Check sheet for the modelled part. Datum: model origin and axes. Units: mm. Coordinates: 2 decimals unless noted, no trailing zeros. Write each loop counter-clockwise with the first axis right and the second up, starting at its lowest first coordinate (ties: lowest second). Pieces come first, ordered by that corner, then holes. Notation, with made-up numbers: (62, 21.5) -> (120, 21.5) arc R36 cw to (120, 55.5) -> close; hole circle Ø8 at (47.25, 37.25). An arc over 180 degrees is marked (long way). Put each result on its own line as item: value.
```python
from build123d import *

# Parameters (mm, degrees)
MODEL_R             = 2.5
MODEL_W             = 7.5
MODEL_H             = 60.000012028
BOSS_EXTRUDE1_DEPTH = 6.35


with BuildPart() as part:
    # Model → Boss-Extrude1 (new body)
    with BuildSketch(Plane.XY):
        Polygon((691.840616937, 302.611489719), (346.840616937, 302.611489719), (346.840616937, 367.611489719), (368.840616937, 367.611489719), (368.840616937, 447.611489719), (345.840616937, 447.611489719), (345.840616937, 534.611489719), (368.840616937, 534.611489719), (368.840616937, 644.611489719), (691.840616937, 644.611489719), align=None)
        with Locations((355.840616937, 514.611489719)):
            Circle(MODEL_R, mode=Mode.SUBTRACT)
        with Locations((355.840616937, 492.611489719)):
            Circle(MODEL_R, mode=Mode.SUBTRACT)
        with Locations((355.840616937, 467.611489719)):
            Circle(MODEL_R, mode=Mode.SUBTRACT)
        with Locations((356.840616937, 347.611489719)):
            Circle(MODEL_R, mode=Mode.SUBTRACT)
        with Locations((356.840616937, 322.611489719)):
            Circle(MODEL_R, mode=Mode.SUBTRACT)
        with Locations((451.840616937, 483.611489719)):
            Circle(MODEL_R, mode=Mode.SUBTRACT)
        with Locations((521.840616937, 483.611489719)):
            Circle(MODEL_R, mode=Mode.SUBTRACT)
        with Locations((601.840616937, 483.611489719)):
            Circle(MODEL_R, mode=Mode.SUBTRACT)
        with Locations((382.628249379, 594.607051385)):
            Rectangle(MODEL_W, MODEL_H, mode=Mode.SUBTRACT)
        Polygon((378.878249379, 382.675054085), (386.377012819, 382.538867187), (386.377012819, 322.632601599), (378.878249379, 322.547926114), align=None, mode=Mode.SUBTRACT)
        Polygon((661.987313401, 624.611489719), (669.487313401, 624.611489719), (669.459063879, 564.611489719), (661.959063879, 564.611489719), align=None, mode=Mode.SUBTRACT)
        Polygon((661.873375206, 382.614770073), (669.373373543, 382.611238884), (669.345124024, 322.611245534), (661.845125687, 322.614776724), align=None, mode=Mode.SUBTRACT)
    extrude(amount=-BOSS_EXTRUDE1_DEPTH)


solid = part.part
```
Q1. Material ranges on line 1 along Y through (x, z) = (384.5, -3); line 2 along X through (y, z) = (380, -2.25); line 3 along X through (y, z) = (624.5, -1), recorded low to high.
Recorded:
line 1: y = 302.61 to 322.61, 382.57 to 564.61, 624.61 to 644.61
line 2: x = 368.84 to 378.88, 386.38 to 661.87, 669.37 to 691.84
line 3: x = 368.84 to 378.88, 386.38 to 661.99, 669.49 to 691.84
Q2. Cross-section at B-B (z = -2.75). State how many separate pieces and enclosed holes the cut face has, plus the area to 3 significant figures.
Recorded:
separate pieces: 1
enclosed holes: 12
area: 112,000 mm2
Q3. Cross-section at A-A (y = 598.5). Record the cut outline in (x, z), plus the area to 3 significant figures.
Recorded:
outline: (368.84, -6.35) -> (378.88, -6.35) -> (378.88, 0) -> (368.84, 0) -> close; (386.38, -6.35) -> (661.98, -6.35) -> (661.98, 0) -> (386.38, 0) -> close; (669.48, -6.35) -> (691.84, -6.35) -> (691.84, 0) -> (669.48, 0) -> close
area: 1,960 mm2
Q4. Depth check by flat-ended pin: P1, Ø3, axis at x = 355.84, y = 492.61, coming from the -Z side; P2, Ø3, axis at y = 346.5, z = -4, coming from the -X side; P3, Ø3, axis at y = 561.5, z = -2, coming from the -X side; P4, Ø3, axis at x = 363, z = -3, coming from the +Y side. Enter the tip coordinate at first touch or a pass-through.
Recorded:
P1: passes through
P2: stops at x = 346.84
P3: stops at x = 368.84
P4: stops at y = 534.61
Q5. Cross-section at C-C (y = 553.5). Record the cut outline in (x, z).
Recorded:
outline: (368.84, -6.35) -> (691.84, -6.35) -> (691.84, 0) -> (368.84, 0) -> close
